from build123d import *

# Parameters (mm, degrees)
F0_W     = 150
F0_H     = 6
F0_W_2   = 6
F0_H_2   = 25
F1_DEPTH = 6
F2_R     = 15
F3_DEPTH = 6


with BuildPart() as f1:
    # F0 (on Right) → F1 (new body)
    with BuildSketch(Plane.YZ):
        Polygon((-75, 25), (-144, 25), (-144, 12.5), (-138, 12.5), (-138, -12.5), (-144, -12.5), (-144, -25), (-75, -25), (-75, -19), (75, -19), (75, -25), (144, -25), (144, -12.5), (138, -12.5), (138, 12.5), (144, 12.5), (144, 25), (75, 25), (75, 19), (-75, 19), align=None)
        with Locations((0, 22)):
            Rectangle(F0_W, F0_H)
        with Locations((0, -28)):
            Rectangle(F0_W, F0_H)
        with Locations((0, -22)):
            Rectangle(F0_W, F0_H)
        with Locations((-141, 0)):
            Rectangle(F0_W_2, F0_H_2)
        with Locations((-147, 0)):
            Rectangle(F0_W_2, F0_H_2)
        with Locations((147, 0)):
            Rectangle(F0_W_2, F0_H_2)
        with Locations((141, 0)):
            Rectangle(F0_W_2, F0_H_2)
    extrude(amount=F1_DEPTH)

    # F2 (on face) → F3 (cut, through all)
    with BuildSketch(Plane.YZ.offset(6)):
        Circle(F2_R)
        with Locations((-80, 0)):
            Circle(F2_R)
        with Locations((80, 0)):
            Circle(F2_R)
    extrude(amount=-F3_DEPTH, mode=Mode.SUBTRACT)


solid = f1.part
For this review, take the finished solid that the model builds, in its own axes (mm). A direction names the side the tool comes from. Give positions to 0.01 mm unless a question says otherwise; leave off trailing zeros. Loops run counter-clockwise (first coordinate to the right, second up) from the corner with the lowest first, then second, coordinate; pieces in that order, holes last. Notation, with made-up numbers: (31, -27) -> (61, -27) arc R28 ccw to (61, 1) -> close; hole circle Ø1 at (64.5, 19). An arc over 180 degrees is marked (long way). One line per question, with ' | ' between items.
1) To check wall thickness, follow probe 1 along Y at (x, z) = (4.15, -1); probe 2 along Y at (x, z) = (5.15, 8.5); probe 3 along Z at (x, y) = (1.8, -80). State the ranges of each line that lie inside material, in increasing order.
Resolved:
probe 1: y = -150 to -94.97, -65.03 to -14.97, 14.97 to 65.03, 94.97 to 150 | probe 2: y = -150 to -92.36, -67.64 to -12.36, 12.36 to 67.64, 92.36 to 150 | probe 3: z = -25 to -15, 15 to 25
2) Insertion check: pin 1 Ø3 at (x, y) = (2.5, -146.5) entering from -Z; pin 2 Ø3 at (x, y) = (2, -97) entering from -Z; pin 3 Ø3 at (x, z) = (4.5, -28.5) entering from +Y. Each pin has a flat end and moves straight along its axis. Give the tip position at first contact, or say it passes through.
Resolved:
pin 1: stops at z = -12.5 | pin 2: stops at z = -25 | pin 3: stops at y = 75
3) We need section D-D (y = 0). Write out the cut boundary in (x, z).
Resolved:
outline: (0, -31) -> (6, -31) -> (6, -15) -> (0, -15) -> close; (0, 15) -> (6, 15) -> (6, 25) -> (0, 25) -> close
4) We need section B-B (z = 9). Write out the cut boundary in (x, y), plus the area to 3 significant figures.
Resolved:
outline: (0, -150) -> (6, -150) -> (6, -92) -> (0, -92) -> close; (0, -68) -> (6, -68) -> (6, -12) -> (0, -12) -> close; (0, 12) -> (6, 12) -> (6, 68) -> (0, 68) -> close; (0, 92) -> (6, 92) -> (6, 150) -> (0, 150) -> close | area: 1,370 mm2
5) We need section A-A (y = -80). Write out the cut boundary in (x, z), plus the area to 3 significant figures.
Resolved:
outline: (0, -25) -> (6, -25) -> (6, -15) -> (0, -15) -> close; (0, 15) -> (6, 15) -> (6, 25) -> (0, 25) -> close | area: 120 mm2
6) We need section C-C (x = 4.5). Write out the cut boundary in (y, z).
Resolved:
outline: (-150, -12.5) -> (-144, -12.5) -> (-144, -25) -> (-75, -25) -> (-75, -31) -> (75, -31) -> (75, -25) -> (144, -25) -> (144, -12.5) -> (150, -12.5) -> (150, 12.5) -> (144, 12.5) -> (144, 25) -> (-144, 25) -> (-144, 12.5) -> (-150, 12.5) -> close; hole circle Ø30 at (-80, 0); hole circle Ø30 at (0, 0); hole circle Ø30 at (80, 0)
7) For faces 4 (the flat face through (3, -147, -12.5)), 5 (the flat face through (3, 147, 12.5)), 6 (the flat face through (3, -147, 12.5)), 7 (the flat face through (3, 144, -19)), list the 3-axis set-ups (+Z, -Z, +X, -X, +Y, -Y) from which the entire face can be reached by the end or side of a thin tool; tool diameter is ignored.
Resolved:
face 4: -Z, +X, -X, -Y | face 5: +Z, +X, -X, +Y | face 6: +Z, +X, -X, -Y | face 7: -Z, +X, -X, +Y
8) The part is to be moulded in two halves that separate along Y. For faces 1 (the flat face through (3, -1, -31)), 2 (the flat face through (3, -144, -19)), 3 (the cylindrical face through (3.042, 65.015, 0.66)), say which applies: +Y half, -Y half, draft (parallel to the pull), parting line (faces both ways), or undercut.
Resolved:
face 1: draft | face 2: -Y half | face 3: undercut
